Verification items for the finished model (mm, model axes). Give positions to 0.01 mm unless a question says otherwise; leave off trailing zeros. Order: outer loops, then holes, each group sorted by start corner. A loop starts at its lowest first (then second) coordinate and runs counter-clockwise, first axis right, second up. Notation, with made-up numbers: (38.25, 29.25) -> (84.25, 29.25) arc R9 cw to (84.25, 41.25) -> close; hole circle Ø1 at (-26, 41). An arc over 180 degrees is marked (long way). Return JSON: item names as keys, results as strings. Group by question number.
(1) Cross-section at C-C on x = -128.5. Enter the section's corners in (y, z).
(2) Depth check by flat-ended pin: pin 1 Ø1 at (x, z) = (-163, 1) entering from -Y; pin 2 Ø3 at (x, y) = (0, 8.5) entering from -Z; pin 3 Ø0.6 at (x, z) = (-172.5, 1) entering from +Y. Enter the tip coordinate at first touch or a pass-through.
(3) Cross-section at A-A on x = -181. Enter the section's corners in (y, z).
(4) Thickness scan on line 1 along Y through (x, z) = (0, 1.1); line 2 along Y through (x, z) = (-60, 1.55); line 3 along X through (y, z) = (2.25, 1). Record the ranges inside material, lowest first.
(5) Cross-section at B-B on z = 0.75. State how many separate pieces and enclosed holes the cut face has, then the cut area to 3 significant figures.
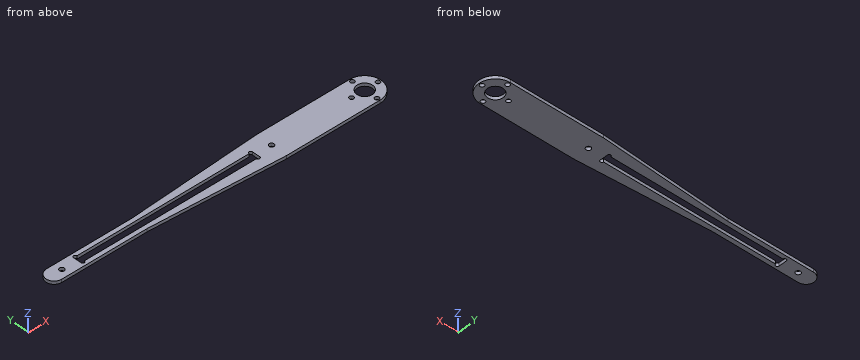
Autodesk Inventor part; units mm, degrees
ref_plane "YZ Plane" through (0, 0, 0) normal (1, 0, 0) x (0, 1, 0)
ref_plane "XZ Plane" through (0, 0, 0) normal (0, 1, 0) x (-1, 0, 0)
ref_plane "XY Plane" through (0, 0, 0) normal (0, 0, 1) x (1, 0, 0)
sketch "スケッチ1" plane through (0, 0, 0) normal (0, 0, 1) x (1, 0, 0)
  circle A0 centre (0, 0) radius 10.5 construction
  line L0 (0, 10.5) -> (-200, 10.5) construction
  line L1 (-200, 10.5) -> (-200, -10.5) construction
  line L2 (-200, -10.5) -> (0, -10.5) construction
  circle A1 centre (-195, 0) radius 1.55
  line L3 (-185, 2.5) -> (-70, 2.5) construction
  line L4 (-70, 2.5) -> (-70, -2.5) construction
  line L5 (-70, -2.5) -> (-185, -2.5) construction
  line L6 (-185, -2.5) -> (-185, 2.5) construction
  line L7 (-127.5, 2.5) -> (-127.5, -2.5) construction
  circle A2 centre (-60, 0) radius 1.55
  line L8 (-12, 21.3027) -> (-12, -27.3903) construction
  line L9 (-69.95, 2.55) -> (-185.05, 2.55) construction
  line L10 (-185.05, 2.55) -> (-185.05, -2.55) construction
  line L11 (-185.05, -2.55) -> (-69.95, -2.55) construction
  line L12 (-69.95, -2.55) -> (-69.95, 2.55) construction
  circle A3 centre (-184, 2.55) radius 1.05 construction
  line L13 (-185, 0) -> (-127.5, 0) construction
  line L14 (-185.05, 2.55) -> (-185.05, -2.55)
  arc A4 (-182.95, 2.55) -> (-185.05, 2.55) centre (-184, 2.55) ccw
  line L15 (-182.95, 2.55) -> (-72.05, 2.55)
  arc A5 (-69.95, 2.55) -> (-72.05, 2.55) centre (-71, 2.55) ccw
  line L16 (-69.95, 2.55) -> (-69.95, -2.55)
  arc A6 (-185.05, -2.55) -> (-182.95, -2.55) centre (-184, -2.55) ccw
  line L17 (-182.95, -2.55) -> (-72.05, -2.55)
  arc A7 (-72.05, -2.55) -> (-69.95, -2.55) centre (-71, -2.55) ccw
  circle A8 centre (0, 8.5) radius 1.35
  circle A9 centre (0, 0) radius 5.05
  circle A10 centre (-8.5, 0) radius 1.35
  circle A11 centre (0, -8.5) radius 1.35
  circle A12 centre (8.5, 0) radius 1.35
  line L18 (-60, 10.5) -> (0, 10.5)
  line L19 (-60, -10.5) -> (0, -10.5)
  arc A13 (0, -10.5) -> (0, 10.5) centre (0, 0) ccw
  circle A14 centre (-195, 0) radius 5 construction
  arc A15 (-200, 5.25) -> (-200, -5.25) centre (-200, 0) ccw
  line L20 (-200, 5.25) -> (-145, 5.25)
  line L21 (-145, 5.25) -> (-60, 10.5)
  line L22 (-200, -5.25) -> (-145, -5.25)
  line L23 (-145, -5.25) -> (-60, -10.5)
  dimension "d9" = 2.1
  dimension "d0" = 200
  dimension "d1" = 3.1
  dimension "d2" = 21
  dimension "d3" = 10
  dimension "d4" = 5
  dimension "d5" = 12
  dimension "d6" = 135
  dimension "d7" = 5
  dimension "d8" = 0.05
  dimension "d10" = 2.7
  dimension "d11" = 8.5
  dimension "d12" = 10.1
  dimension "d15" = 360
  dimension "d20" = 5.25
  dimension "d21" = 50
extrude "押し出し1" add sketch "スケッチ1" along normal blind 2
fillet "フィレット1" radius 2 2 edges at (-145, -5.25, 1) (-145, 5.25, 1)
equation "\"H_head\" = 28.5"
equation "\"H_leg\" = 199.5"
equation "\"足の面積\" = 12720.125"
equation "\"現在の面積\" = 11560"
equation "\"足_短辺\" = 68"
equation "\"円柱\" = 313.5"
equation "\"胴体中心から手先\" = 342"
equation "\"H_leg_1\" = 186.2"
equation "\"H_leg_MAX\" = 399"
equation "\"H_head_1\" = 26.6"
equation "\"H_head_MAX\" = 142.5"
properties part number "ForeArm_outside_frame" material "GFRP"
Verdict:
{
 "1": {"outline": "(-6.27, 0) -> (-2.55, 0) -> (-2.55, 2) -> (-6.27, 2) -> close; (2.55, 0) -> (6.27, 0) -> (6.27, 2) -> (2.55, 2) -> close"},
 "2": {"pin 1": "y = -5.25", "pin 2": "z = 0", "pin 3": "y = 5.25"},
 "3": {"outline": "(-5.25, 0) -> (-2.55, 0) -> (-2.55, 2) -> (-5.25, 2) -> close; (2.55, 0) -> (5.25, 0) -> (5.25, 2) -> (2.55, 2) -> close"},
 "4": {"line 1": "-10.5 to -9.85, -7.15 to -5.05, 5.05 to 7.15, 9.85 to 10.5", "line 2": "-10.5 to -1.55, 1.55 to 10.5", "line 3": "-204.74 to -185.05, -69.95 to -4.52, 4.52 to 10.26"},
 "5": {"separate pieces": "1", "enclosed holes": "8", "area": "2,680 mm²"}
}
